Geometry: final body of the model. Coordinates: model frame, mm. Round coordinates to 2 decimals unless told otherwise and drop trailing zeros. Loops run counter-clockwise (first coordinate to the right, second up) from the corner with the lowest first, then second, coordinate; pieces in that order, holes last. Notation, with made-up numbers: (-29, 62) -> (-16, 62) arc R15 ccw to (-16, 74) -> close; hole circle Ø10 at (35, -18.5). An arc over 180 degrees is marked (long way). Answer in a Markdown table with one row per item.
```python
from build123d import *

# Parameters (mm, degrees)
CROQUIS1_R            = 27.5
BRIDA_BASE1_DEPTH     = 0.5
CROQUIS6_R            = 11.25
CROQUIS6_R_2          = 1.5
CORTAR_EXTRUIR3_DEPTH = 10


# Sheet-metal steps are written as plain solids
with BuildPart() as part:
    # Croquis1 → Brida base1 (new body)
    with BuildSketch(Plane.XY):
        Circle(CROQUIS1_R)
    extrude(amount=-BRIDA_BASE1_DEPTH)

    # Croquis6 → Cortar-Extruir3 (cut)
    with BuildSketch(Plane.XY):
        Circle(CROQUIS6_R)
        with Locations((-13, 13)):
            Circle(CROQUIS6_R_2)
        with Locations((-13, -13)):
            Circle(CROQUIS6_R_2)
        with Locations((13, 13)):
            Circle(CROQUIS6_R_2)
        with Locations((0, 25)):
            Circle(CROQUIS6_R_2)
        with Locations((-15.5, 15.5)):
            Circle(CROQUIS6_R_2)
        with Locations((-15.5, -15.5)):
            Circle(CROQUIS6_R_2)
        with Locations((0, -25)):
            Circle(CROQUIS6_R_2)
        with Locations((13, -13)):
            Circle(CROQUIS6_R_2)
        with Locations((15.5, -15.5)):
            Circle(CROQUIS6_R_2)
        with Locations((15.5, 15.5)):
            Circle(CROQUIS6_R_2)
    extrude(amount=-CORTAR_EXTRUIR3_DEPTH, mode=Mode.SUBTRACT)


solid = part.part
```
Item 1: Cut plane A-A (x = 0). Output: boundary loops of the cut face in (y, z), then the cut area to 4 significant figures.
Answer:
| item | result |
|---|---|
| outline | (-27.5, -0.5) -> (-26.5, -0.5) -> (-26.5, 0) -> (-27.5, 0) -> close; (-23.5, -0.5) -> (-11.25, -0.5) -> (-11.25, 0) -> (-23.5, 0) -> close; (11.25, -0.5) -> (23.5, -0.5) -> (23.5, 0) -> (11.25, 0) -> close; (26.5, -0.5) -> (27.5, -0.5) -> (27.5, 0) -> (26.5, 0) -> close |
| area | 13.25 mm² |
Item 2: Cut plane B-B (y = 0). Output: boundary loops of the cut face in (x, z), then the cut area to 4 significant figures.
Answer:
| item | result |
|---|---|
| outline | (-27.5, -0.5) -> (-11.25, -0.5) -> (-11.25, 0) -> (-27.5, 0) -> close; (11.25, -0.5) -> (27.5, -0.5) -> (27.5, 0) -> (11.25, 0) -> close |
| area | 16.25 mm² |
Item 3: Pin query (flat end, axial travel): pin 1 Ø1.8 at (x, y) = (13, 13) entering from +Z. Return the tip coordinate at first contact, or that it passes through.
Answer:
| item | result |
|---|---|
| pin 1 | passes through |
Item 4: Cut plane C-C (z = -0.2). Count the separate pieces of the cut face and the enclosed holes in it, then the cut area to 3 significant figures.
Answer:
| item | result |
|---|---|
| separate pieces | 1 |
| enclosed holes | 11 |
| area | 1,910 mm² |
Item 5: Line query: probe 1 along Y at (x, z) = (0, -0.3); probe 2 along Y at (x, z) = (-13.5, -0.35); probe 3 along Y at (x, z) = (13, -0.15). Output: solid intervals per line, ascending. Write a range as [from, to].
Answer:
| item | result |
|---|---|
| probe 1 | y = [-27.5, -26.5], [-23.5, -11.25], [11.25, 23.5], [26.5, 27.5] |
| probe 2 | y = [-23.96, -14.41], [-11.59, 11.59], [14.41, 23.96] |
| probe 3 | y = [-24.23, -14.5], [-11.5, 11.5], [14.5, 24.23] |
Item 6: Cut plane D-D (y = -15.5). Output: boundary loops of the cut face in (x, z), then the cut area to 3 significant figures.
Answer:
| item | result |
|---|---|
| outline | (-22.72, -0.5) -> (-17, -0.5) -> (-17, 0) -> (-22.72, 0) -> close; (-14, -0.5) -> (14, -0.5) -> (14, 0) -> (-14, 0) -> close; (17, -0.5) -> (22.72, -0.5) -> (22.72, 0) -> (17, 0) -> close |
| area | 19.7 mm² |
Item 7: Draft query along Y for faces 1 (the face through (0, -12, 0)), 2 (the face through (-5.961, -26.846, -0.246)), 3 (the face through (14, 15.57, -0.25)). Return one class per face: pulls with the +Y half, pulls with the -Y half, needs draft (parallel to the pull), parting line crosses it, or undercut.
Answer:
| item | result |
|---|---|
| face 1 | needs draft |
| face 2 | parting line crosses it |
| face 3 | undercut |
